Read the model definition and answer for the solid it produces. Units are mm, in the model's axes. Face numbers are marked on the shaded views. A direction names the side the tool comes from. Round coordinates to 2 decimals unless told otherwise and drop trailing zeros. Loops run counter-clockwise (first coordinate to the right, second up) from the corner with the lowest first, then second, coordinate; pieces in that order, holes last. Notation, with made-up numbers: (40, 60.25) -> (98, 60.25) arc R15 ccw to (98, 89.25) -> close; hole circle Ø7 at (49.5, 49). An arc over 180 degrees is marked (long way). Put each result on its own line as item: value.
from build123d import *
from build123d.topology import SkipClean

# Parameters (mm, degrees)
SCHIZZO1_R                   = 1.75
SCHIZZO1_R_2                 = 12.5
ESTRUSIONE_ESTRUSIONE1_DEPTH = 3
ESTRUSIONE_ESTRUSIONE2_DEPTH = 10
SCHIZZO3_R                   = 3
ESTRUSIONE_ESTRUSIONE3_DEPTH = 2.2


with BuildPart() as part:
    # Schizzo1 → Estrusione-Estrusione1 (new body)
    # profile 1 of 3: a face of its own
    with SkipClean():  # the faces are left unmerged after this step: merging them gives an invalid solid
        with BuildSketch(Plane.XY):
            with BuildLine():
                Line((-8.291561976, 12.5), (-25, 12.5))
                Line((-25, 12.5), (-25, -25))
                Line((-25, -25), (25, -25))
                Line((25, -25), (25, 12.5))
                Line((25, 12.5), (8.291561976, 12.5))
                ThreePointArc((8.291561976, 12.5), (0, -15), (-8.291561976, 12.5))
            make_face()
            with Locations((-20, -21.25)):
                Circle(SCHIZZO1_R, mode=Mode.SUBTRACT)
            with Locations((20, -21.25)):
                Circle(SCHIZZO1_R, mode=Mode.SUBTRACT)
            with Locations((-20, 8.75)):
                Circle(SCHIZZO1_R, mode=Mode.SUBTRACT)
            with Locations((20, 8.75)):
                Circle(SCHIZZO1_R, mode=Mode.SUBTRACT)
        # profile 2 of 3: a face of its own
        with BuildSketch(Plane.XY):
            with BuildLine():
                Line((-4.8e-08, 12.5), (-8.291561976, 12.5))
                ThreePointArc((-8.291561976, 12.5), (0, -15), (8.291561976, 12.5))
                Line((8.291561976, 12.5), (-4.8e-08, 12.5))
            make_face()
            with BuildLine():
                ThreePointArc((12.5, 0), (-8.838834748, -8.838834782), (-4.8e-08, 12.5))
                ThreePointArc((-4.8e-08, 12.5), (8.838834748, 8.838834782), (12.5, 0))
            make_face(mode=Mode.SUBTRACT)
        # profile 3 of 3: a face of its own
        with BuildSketch(Plane.XY):
            Circle(SCHIZZO1_R_2)
            Circle(SCHIZZO1_R, mode=Mode.SUBTRACT)
        extrude(amount=ESTRUSIONE_ESTRUSIONE1_DEPTH)

    # Schizzo2 → Estrusione-Estrusione2 (add)
    with BuildSketch(Plane.XY.offset(3)):
        with BuildLine():
            Line((15, 0), (15, 12.5))
            Line((15, 12.5), (12.5, 12.5))
            Line((12.5, 12.5), (12.5, 0))
            ThreePointArc((12.5, 0), (0, -12.5), (-12.5, 0))
            Line((-12.5, 0), (-12.5, 12.5))
            Line((-12.5, 12.5), (-15, 12.5))
            Line((-15, 12.5), (-15, 0))
            ThreePointArc((-15, 0), (0, -15), (15, 0))
        make_face()
    extrude(amount=ESTRUSIONE_ESTRUSIONE2_DEPTH)

    # Schizzo3 → Estrusione-Estrusione3 (add)
    with BuildSketch(Plane.XY.offset(3)):
        with BuildLine():
            Line((12.5, 0), (12.5, 12.5))
            Line((12.5, 12.5), (-12.5, 12.5))
            Line((-12.5, 12.5), (-12.5, 0))
            ThreePointArc((-12.5, 0), (0, -12.5), (12.5, 0))
        make_face()
        Circle(SCHIZZO3_R, mode=Mode.SUBTRACT)
    extrude(amount=ESTRUSIONE_ESTRUSIONE3_DEPTH)


solid = part.part
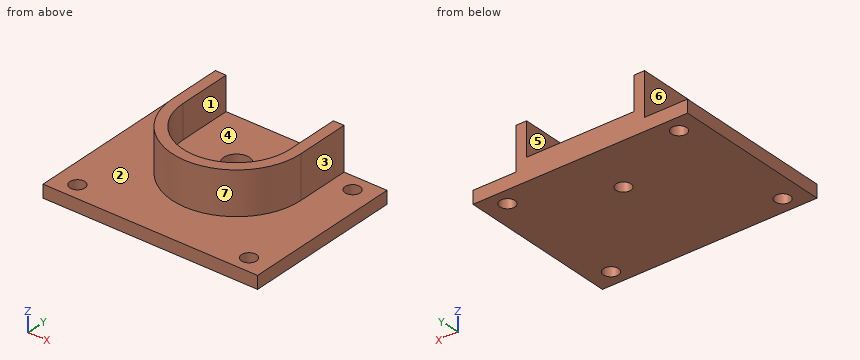
Item 1: Flat-ended cylindrical pins translate along their axes: pin 1 Ø4 at (y, z) = (6.5, 10.5) entering from -X; pin 2 Ø1.5 at (x, z) = (-11, 4.5) entering from -Y; pin 3 Ø3 at (y, z) = (6.5, 7) entering from +X. Find the tip coordinate at first contact, or state that the pin passes through.
Derived:
pin 1: stops at x = -15
pin 2: stops at y = -10.95
pin 3: stops at x = 15
Item 2: The part is cut by section C-C (z = 11.25). Determine the outline of the cut face in (x, y).
Derived:
outline: (-15, 0) arc R15 ccw to (15, 0) -> (15, 12.5) -> (12.5, 12.5) -> (12.5, 0) arc R12.5 cw to (-12.5, 0) -> (-12.5, 12.5) -> (-15, 12.5) -> close
Item 3: Find the intervals of material crossed by line 1 along Y through (x, z) = (-20, 0.85); line 2 along Y through (x, z) = (0, 1.4); line 3 along Y through (x, z) = (0, 4.05), in increasing order.
Derived:
line 1: y = -25 to -23, -19.5 to 7, 10.5 to 12.5
line 2: y = -25 to -1.75, 1.75 to 12.5
line 3: y = -15 to -3, 3 to 12.5
Item 4: The part is cut by section A-A (y = -21.25). Determine the outline of the cut face in (x, z), then the cut area to 3 significant figures.
Derived:
outline: (-25, 0) -> (-21.75, 0) -> (-21.75, 3) -> (-25, 3) -> close; (-18.25, 0) -> (18.25, 0) -> (18.25, 3) -> (-18.25, 3) -> close; (21.75, 0) -> (25, 0) -> (25, 3) -> (21.75, 3) -> close
area: 129 mm^2
Item 5: Which of the six approach directions +Z, -Z, +X, -X, +Y, -Y give full straight-line access (tool end or side, diameter ignored) to the marked faces 5, 6 and 7?
Derived:
face 5: +Z, +Y
face 6: +Z, -X, +Y, -Y
face 7: +Z, -Y
Item 6: The part is cut by section B-B (x = 0). Determine the outline of the cut face in (y, z), then the cut area to 3 significant figures.
Derived:
outline: (-25, 0) -> (-1.75, 0) -> (-1.75, 3) -> (-3, 3) -> (-3, 5.2) -> (-12.5, 5.2) -> (-12.5, 13) -> (-15, 13) -> (-15, 3) -> (-25, 3) -> close; (1.75, 0) -> (12.5, 0) -> (12.5, 5.2) -> (3, 5.2) -> (3, 3) -> (1.75, 3) -> close
area: 169 mm^2
Item 7: For a pull along X with two mould halves and no side action, classify the marked faces 1, 2, 3 and 4 as pulls with the +X half, pulls with the -X half, needs draft (parallel to the pull), parting line crosses it, or undercut.
Derived:
face 1: undercut
face 2: needs draft
face 3: pulls with the +X half
face 4: undercut
Item 8: The part is cut by section D-D (x = 20). Determine the outline of the cut face in (y, z).
Derived:
outline: (-25, 0) -> (-23, 0) -> (-23, 3) -> (-25, 3) -> close; (-19.5, 0) -> (7, 0) -> (7, 3) -> (-19.5, 3) -> close; (10.5, 0) -> (12.5, 0) -> (12.5, 3) -> (10.5, 3) -> close
